The listing builds one solid part. Answer for the finished solid, in the listing's coordinates (mm). Face numbers are marked on the shaded views. Coordinates: 2 decimals unless noted, no trailing zeros. Order: outer loops, then holes, each group sorted by start corner. A loop starts at its lowest first (then second) coordinate and runs counter-clockwise, first axis right, second up. Notation, with made-up numbers: (-1, -3) - (11, -3) arc R5 ccw to (11, 4) - close; hole circle Ø11 at (9.25, -32.75). An arc over 180 degrees is marked (long way). Use one line per item in the form item = value. Start each with the question number.
Item 1: The mould has two halves that part along Z. Classify the marked faces 1, 2 and 3: released by +Z, released by -Z, zero draft, split by the parting line, or undercut.
Item 2: Section C-C, the plane z = 16 is taken. Write down the section's boundary in (x, y).
Item 3: Each of these flat-tipped pins is pushed along its axis until it touches: pin 1 Ø2 at (x, y) = (-16, 4.5) entering from +Z; pin 2 Ø2.5 at (y, z) = (4.5, 13) entering from +X; pin 3 Ø1.5 at (x, z) = (-1.5, 12) entering from +Y. Where does it stop, or does it pass through?
Item 4: Section D-D, the plane x = -4 is taken. Write down the section's boundary in (y, z), and give its area (3 significant figures).
Item 5: Section A-A, the plane x = -21 is taken. Write down the section's boundary in (y, z), and give its area (3 significant figures).
Item 6: Section B-B, the plane y = 3.3 is taken. Write down the section's boundary in (x, z).
Item 7: Consider line 1 along X through (y, z) = (1.8, 21.5); line 2 along Y through (x, z) = (11, 2.5); line 3 along Z through (x, y) = (-16, 3.8). Determine where each line is inside the solid, lowest interval first. Write a range as [from, to].
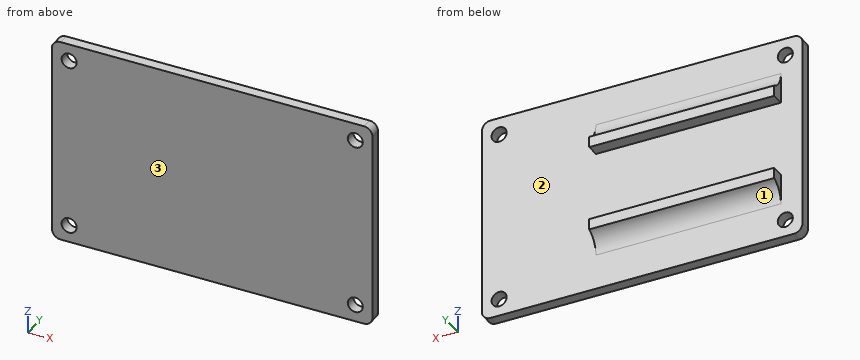
from build123d import *

# Parameters (mm, degrees)
SKETCH1_R           = 1.75
BOSS_EXTRUDE1_DEPTH = 2.5
SKETCH2_W           = 43
SKETCH2_H           = 2.5
BOSS_EXTRUDE2_DEPTH = 3
FILLET1_R           = 5


with BuildPart() as part:
    # Sketch1 → Boss-Extrude1 (new body)
    with BuildSketch(Plane(origin=(0, 0, 0), x_dir=(1, 0, 0), z_dir=(0, 1, 0))):
        with BuildLine():
            Line((-52.476274799, 21.3340289), (18.023725201, 21.3340289))
            ThreePointArc((18.023725201, 21.3340289), (19.437938764, 20.748242463), (20.023725201, 19.3340289))
            Line((20.023725201, 19.3340289), (20.023725201, -24.6659711))
            ThreePointArc((20.023725201, -24.6659711), (19.437938764, -26.080184662), (18.023725201, -26.6659711))
            Line((18.023725201, -26.6659711), (-52.476274799, -26.6659711))
            ThreePointArc((-52.476274799, -26.6659711), (-53.890488361, -26.080184662), (-54.476274799, -24.6659711))
            Line((-54.476274799, -24.6659711), (-54.476274799, 19.3340289))
            ThreePointArc((-54.476274799, 19.3340289), (-53.890488361, 20.748242463), (-52.476274799, 21.3340289))
        make_face()
        with Locations(Location((-50.476274799, 17.3340289, 0), (0, 0, 270))):
            Circle(SKETCH1_R, mode=Mode.SUBTRACT)
        with Locations(Location((16.023725201, 17.3340289, 0), (0, 0, 270))):
            Circle(SKETCH1_R, mode=Mode.SUBTRACT)
        with Locations(Location((16.023725201, -22.6659711, 0), (0, 0, 270))):
            Circle(SKETCH1_R, mode=Mode.SUBTRACT)
        with Locations(Location((-50.476274799, -22.6659711, 0), (0, 0, 270))):
            Circle(SKETCH1_R, mode=Mode.SUBTRACT)
    extrude(amount=BOSS_EXTRUDE1_DEPTH)

    # Sketch2 → Boss-Extrude2 (add)
    with BuildSketch(Plane(origin=(0, 2.5, 0), x_dir=(1, 0, 0), z_dir=(0, 1, 0))):
        with Locations((-27.976274799, 7.3340289)):
            Rectangle(SKETCH2_W, SKETCH2_H)
        with Locations((-27.976274799, -12.6659711)):
            Rectangle(SKETCH2_W, SKETCH2_H)
    extrude(amount=BOSS_EXTRUDE2_DEPTH)

    # Fillet1
    # the kernel refuses this fillet: 5 mm, written as the material it adds along each edge
    with BuildSketch(Plane(origin=(-49.476274799, 2.5, -8.5840289), x_dir=(0, 0, -1), z_dir=(1, 0, 0)), Plane(origin=(-6.476274799, 2.5, 13.9159711), x_dir=(0, 0, 1), z_dir=(-1, 0, 0))) as fillet1_piece_1:
        with BuildLine():
            CenterArc((4.582575695, 5), FILLET1_R, 203.578178478, 66.421821522)
            Line((0, 3), (-0.091651514, 2.96))
            ThreePointArc((-0.091651514, 2.96), (-0.1, 1.5), (-0.1, 0))
            Line((-0.1, 0), (0, -0.1))
            Line((0, -0.1), (4.582575695, -0.1))
            Line((4.582575695, -0.1), (4.582575695, 0))
        make_face()
    extrude(amount=43)


solid = part.part
Response:
q1.face_1 = released by -Z
q1.face_2 = undercut
q1.face_3 = zero draft
q2.outline = (-54.48, 0) - (20.02, 0) - (20.02, 2.5) - (-6.48, 2.5) - (-6.48, 3.17) - (-49.48, 3.17) - (-49.48, 2.5) - (-54.48, 2.5) - close
q3.pin_1 = 15.5
q3.pin_2 = -6.48
q3.pin_3 = 2.5
q4.outline = (0, -21.33) - (2.5, -21.33) - (2.5, 26.67) - (0, 26.67) - close
q4.area = 120 mm2
q5.outline = (0, -21.33) - (2.5, -21.33) - (2.5, -13.17) arc R5 cw to (5.5, -8.58) - (5.5, -6.08) - (2.5, -6.08) - (2.5, 11.42) - (5.5, 11.42) - (5.5, 13.92) arc R5 cw to (2.5, 18.5) - (2.5, 26.67) - (0, 26.67) - close
q5.area = 143 mm2
q6.outline = (-49.48, -10.45) - (-6.48, -10.45) - (-6.48, -6.08) - (-49.48, -6.08) - close; (-49.48, 11.42) - (-6.48, 11.42) - (-6.48, 15.79) - (-49.48, 15.79) - close
q7.line_1 = [-54.48, -51.78], [-49.17, 14.72], [17.33, 20.02]
q7.line_2 = [0, 2.5]
q7.line_3 = [-9.8, -6.08], [11.42, 15.14]
